Build history of the part. All positions in model axes, mm. A direction names the side the tool comes from. Round coordinates to 2 decimals unless told otherwise and drop trailing zeros. Write each loop counter-clockwise with the first axis right and the second up, starting at its lowest first coordinate (ties: lowest second). Pieces come first, ordered by that corner, then holes. Notation, with made-up numbers: (80.5, -10.75) -> (122.5, -10.75) arc R32 cw to (122.5, 23.25) -> close; hole circle Ø4 at (-5.5, 38.5). An arc over 180 degrees is marked (long way). Answer as CSV lines item,"result".
from build123d import *

# Parameters (mm, degrees)
SKETCH1_W           = 38.1
SKETCH1_H           = 1.5875
BOSS_EXTRUDE1_DEPTH = 25.4
SKETCH2_W           = 15.875
SKETCH2_H           = 10.16
CUT_EXTRUDE1_DEPTH  = 25.4


with BuildPart() as part:
    # Sketch1 → Boss-Extrude1 (new body)
    with BuildSketch(Plane(origin=(0, 0, 0), x_dir=(1, 0, 0), z_dir=(0, 1, 0))):
        Polygon((26.476413323, 23.684114825), (24.888913323, 23.684114825), (24.888913323, -8.065885175), (24.888913323, -9.653385175), (26.476413323, -9.653385175), align=None)
        with Locations((5.838913323, -8.859635175)):
            Rectangle(SKETCH1_W, SKETCH1_H)
        Polygon((-13.211086677, -9.653385175), (-13.211086677, -8.065885175), (-14.798586677, -8.065885175), (-14.798586677, -23.940885175), (-13.211086677, -23.940885175), align=None)
    extrude(amount=BOSS_EXTRUDE1_DEPTH)

    # Sketch2 → Cut-Extrude1 (cut)
    with BuildSketch(Plane(origin=(26.476413323, 0, 0), x_dir=(0, 0, -1), z_dir=(1, 0, 0))):
        with Locations((15.746614825, 12.7)):
            Rectangle(SKETCH2_W, SKETCH2_H)
    extrude(amount=-CUT_EXTRUDE1_DEPTH, mode=Mode.SUBTRACT)


solid = part.part
1. Probe line 1 along Z through (x, y) = (25, 12.25); line 2 along Z through (x, y) = (0, 9.25); line 3 along X through (y, z) = (5.75, -6). List the from-to ranges inside material, lowest first.
Results found:
line 1,"z = -7.81 to 9.65"
line 2,"z = 8.07 to 9.65"
line 3,"x = 24.89 to 26.48"
2. Which spindle directions (+Z, -Z, +X, -X, +Y, -Y) get a long thin tool onto all of the face, cutting with end or side? Do faces 5 (the flat face through (26, 13, -7.809)), 6 (the flat face through (6, 13, 9.653)), 7 (the flat face through (5, 13, 8.066)). Say none if no direction does.
Results found:
face 5,"-Z, +X, -X"
face 6,"+Z, +X, +Y, -Y"
face 7,"-Z, -X, +Y, -Y"
3. Cut at C-C, the plane x = 13. Write the cut outline in (y, z).
Results found:
outline,"(0, 8.07) -> (25.4, 8.07) -> (25.4, 9.65) -> (0, 9.65) -> close"
4. Cut at D-D, the plane z = -3. Write the cut outline in (x, y), then the cut area to 3 significant figures.
Results found:
outline,"(24.89, 0) -> (26.48, 0) -> (26.48, 25.4) -> (24.89, 25.4) -> close"
area,"40.3 mm2"
5. Cut at A-A, the plane z = -17. Write the cut outline in (x, y).
Results found:
outline,"(24.89, 0) -> (26.48, 0) -> (26.48, 7.62) -> (24.89, 7.62) -> close; (24.89, 17.78) -> (26.48, 17.78) -> (26.48, 25.4) -> (24.89, 25.4) -> close"
6. Cut at B-B, the plane y = 6.5. Write the cut outline in (x, z).
Results found:
outline,"(-14.8, 8.07) -> (24.89, 8.07) -> (24.89, -23.68) -> (26.48, -23.68) -> (26.48, 9.65) -> (-13.21, 9.65) -> (-13.21, 23.94) -> (-14.8, 23.94) -> close"
7. Mould opens along Y. For faces 1 (the flat face through (26, 7.62, -16)), 2 (the flat face through (9, 25.4, 9)), 3 (the flat face through (-13.211, 13, 17)), 4 (the flat face through (9, 0, 9)) say: +Y half, -Y half, draft (parallel to the pull), parting line (faces both ways), or undercut.
Results found:
face 1,"undercut"
face 2,"+Y half"
face 3,"draft"
face 4,"-Y half"
8. Drop flat-ended pins along their axis: pin 1 Ø0.5 at (x, y) = (25.5, 10.5) entering from -Z; pin 2 Ø4 at (x, z) = (11.5, 11) entering from -Y; pin 3 Ø4.5 at (y, z) = (10, 20) entering from +X; pin 4 Ø1 at (x, y) = (4.5, 6.5) entering from +Z. Give the stop position or say it passes through.
Results found:
pin 1,"stops at z = -7.81"
pin 2,"stops at y = 0"
pin 3,"stops at x = -13.21"
pin 4,"stops at z = 9.65"
